Work out the finished part from the listing and answer in its coordinate system (mm). A direction names the side the tool comes from. Coordinates: 2 decimals unless noted, no trailing zeros. Order: outer loops, then holes, each group sorted by start corner. A loop starts at its lowest first (then second) coordinate and runs counter-clockwise, first axis right, second up.
1. A tool of negligible diameter and unlimited length cuts with its end or side. For faces 5 (the flat face through (10, -17, -17)), 6 (the cylindrical face through (18.11, 20.6, 12.68)), 7 (the flat face through (36, 2, -2)), from which of +Z, -Z, +X, -X, +Y, -Y can it reach the whole face along a straight path? Write none if from no direction.
2. Find the intervals of material crossed by probe 1 along Y at (x, z) = (33.5, 15.75); probe 2 along Z at (x, y) = (31, 15); probe 3 along X at (y, z) = (-17, -3.5), in increasing order.
3. Flat-ended cylindrical pins translate along their axes: pin 1 Ø4.5 at (y, z) = (-14.5, 15.5) entering from +X; pin 2 Ø2.5 at (x, z) = (44.5, 0) entering from +Y; pin 3 Ø1.8 at (y, z) = (15.75, 15.75) entering from +X. Find the tip coordinate at first contact, or state that the pin passes through.
4. The part is cut by section C-C, the plane x = 19.5. Give the vertices of the cut face in (y, z), then the cut area to 3 significant figures.
5. Determine the mould class of faces 1 (the cylindrical face through (32.06, -15.68, 17.25)), 2 (the flat face through (17.9, -16.8, -16.7)), 3 (the flat face through (28, -16, -16)), 4 (the cylindrical face through (18.11, -12.68, 20.6)) for opening direction Z: +Z half, -Z half, draft (parallel to the pull), parting line (faces both ways), or undercut.
6. The part is cut by section B-B, the plane z = 0. Give the vertices of the cut face in (x, y), then the cut area to 3 significant figures.
7. The part is cut by section A-A, the plane y = 15.75. Give the vertices of the cut face in (x, z), then the cut area to 3 significant figures.
Autodesk Inventor part; units mm, degrees
ref_plane "YZ Plane" through (0, 0, 0) normal (1, 0, 0) x (0, 1, 0)
ref_plane "XZ Plane" through (0, 0, 0) normal (0, 1, 0) x (-1, 0, 0)
ref_plane "XY Plane" through (0, 0, 0) normal (0, 0, 1) x (1, 0, 0)
sketch "Skizze2" plane through (0, 0, 0) normal (1, 0, 0) x (0, 1, 0)
  line L0 (20.75, -20.75) -> (-20.75, -20.75)
  line L1 (-20.75, -20.75) -> (-20.75, 20.75)
  line L2 (-20.75, 20.75) -> (20.75, 20.75)
  line L3 (20.75, 20.75) -> (20.75, -20.75)
  line L4 (-29.05, 0) -> (29.05, 0)
  line L5 (0, -29.05) -> (0, 29.05)
  point P0 (0, 0)
  dimension "d0" = 41.5
  dimension "d1" = 41.5
extrude "Extrusion1" add sketch "Skizze2" along normal blind 10
chamfer "Fase1" distance 3.5 angle 45 4 edges at (5, 20.75, 20.75) (5, 20.75, -20.75) (5, -20.75, -20.75) (5, -20.75, 20.75)
sketch "Skizze5" plane through (10, 0, 0) normal (1, 0, 0) x (0, 0, -1)
  line L0 (20.75, 20.75) -> (-20.75, 20.75)
  line L1 (-20.75, 20.75) -> (-20.75, -20.75)
  line L2 (-20.75, -20.75) -> (20.75, -20.75)
  line L3 (20.75, -20.75) -> (20.75, 20.75)
  line L4 (0, -29.064) -> (0, 29.1338)
  line L5 (17.25, 20.75) -> (-17.25, 20.75)
  line L6 (29.05, 0) -> (-29.05, 0)
  line L7 (20.75, -17.25) -> (20.75, 17.25)
  line L8 (20.75, 12.75) -> (12.75, 20.75)
  line L9 (17.25, 20.75) -> (20.75, 17.25)
  line L10 (-12.75, 20.75) -> (-20.75, 12.75)
  line L11 (-20.75, -12.75) -> (-12.75, -20.75)
  line L12 (12.75, -20.75) -> (20.75, -12.75)
  point P0 (0, 0)
  dimension "d11" = 41.5
  dimension "d12" = 41.5
  dimension "d20" = 8
  dimension "d21" = 8
  dimension "d24" = 360
extrude "Extrusion5" add sketch "Skizze5" along normal blind 16 contours L8 L3 L6 L4 L0 | L4 L6 L1 L10 L0 | L3 L12 L2 L4 L6 | L4 L2 L11 L1 L6
sketch "Skizze6" plane through (26, 0, 0) normal (1, 0, 0) x (0, 0, -1)
  line L0 (20.75, 20.75) -> (-20.75, 20.75)
  line L1 (-20.75, 20.75) -> (-20.75, -20.75)
  line L2 (-20.75, -20.75) -> (20.75, -20.75)
  line L3 (20.75, -20.75) -> (20.75, 20.75)
  line L4 (29.05, 0) -> (-29.05, 0)
  line L5 (0, -29.05) -> (0, 29.05)
  line L6 (20.75, 12.75) -> (20.75, 17.25)
  line L7 (20.75, 17.25) -> (17.25, 20.75)
  line L8 (-17.25, 20.75) -> (-20.75, 17.25)
  line L9 (-20.75, -17.25) -> (-17.25, -20.75)
  line L10 (17.25, -20.75) -> (20.75, -17.25)
  point P0 (0, 0)
  dimension "d28" = 41.5
  dimension "d29" = 41.5
  dimension "d32" = 360
extrude "Extrusion6" add sketch "Skizze6" along normal blind 10 contours L7 L3 L4 L5 L0 | L5 L4 L1 L8 L0 | L5 L2 L9 L1 L4 | L4 L3 L10 L2 L5
fillet "Rundung1" radius 2 8 edges at (18, 12.75, -20.75) (18, 20.75, -12.75) (18, -12.75, -20.75) (18, -20.75, -12.75) (18, -20.75, 12.75) (18, -12.75, 20.75) (18, 12.75, 20.75) (18, 20.75, 12.75)
sketch "Skizze7" plane through (36, 0, 0) normal (1, 0, 0) x (0, 0, -1)
  circle A0 centre (0, 0) radius 11.5
  circle A1 centre (15.75, -15.75) radius 1.5
  circle A2 centre (15.75, 15.75) radius 1.5
  circle A3 centre (-15.75, -15.75) radius 1.5
  circle A4 centre (-15.75, 15.75) radius 1.5
  dimension "d37" = 23
  dimension "d61" = 3
  dimension "d62" = 3
  dimension "d67" = 15.75
  dimension "d68" = 15.75
  dimension "d69" = 3
  dimension "d70" = 3
  dimension "d71" = 15.75
  dimension "d72" = 15.75
extrude "Extrusion7" add sketch "Skizze7" along normal blind 2 contours A0
sketch "Skizze8" plane through (38, 0, 0) normal (1, 0, 0) x (0, 0, -1)
  circle A0 centre (0, 0) radius 4
  dimension "d40" = 8
extrude "Extrusion8" cut sketch "Skizze8" against normal blind 2
sketch "Skizze9" plane through (36, 0, 0) normal (1, 0, 0) x (0, 0, -1)
  circle A0 centre (0, 0) radius 2.5
  line L0 (2.5, 0) -> (-2.5, 0)
  line L1 (-2.5, 0) -> (-2.5, 2.5)
  line L2 (-2.5, 2.5) -> (2.5, 2.5)
  line L3 (2.5, 2.5) -> (2.5, 0)
  line L4 (2.5, 2.5) -> (-2.5, 2.5)
  line L5 (-2.5, 2.5) -> (-2.5, 2)
  line L6 (-2.5, 2) -> (2.5, 2)
  line L7 (2.5, 2) -> (2.5, 2.5)
  point P0 (1.5, 2)
  point P1 (-1.5, 2)
  dimension "d43" = 5
  dimension "d44" = 0.5
  dimension "d47" = 2
extrude "Extrusion9" add sketch "Skizze9" along normal blind 20 contours L0 A0 | A0 L6 L0
sketch "Skizze10" plane through (0, -20.75, -17.25) normal (0, -1, 0) x (1, 0, 0)
  line L0 (0, 0) -> (0, 34.5)
  line L1 (0, 24.75) -> (10, 24.75)
  line L2 (10, 24.75) -> (10, 9.75)
  line L3 (10, 9.75) -> (0, 9.75)
  line L4 (0, 9.75) -> (0, 24.75)
  line L5 (0, 17.25) -> (36, 17.25)
  line L6 (36, 34.5) -> (36, 0)
  dimension "d48" = 10
  dimension "d49" = 15
extrude "Extrusion10" add sketch "Skizze10" along normal blind 4
extrude "Extrusion11" cut sketch "Skizze7" against normal blind 8 contours A1 | A2 | A3 | A4
properties part number "Steppermotor"
Geometry says:
1. face 5: -Z, -Y
1. face 6: +Z, +Y
1. face 7: +X
2. probe 1: y = -20.75 to -17.25, -14.25 to 14.25, 17.25 to 20.75
2. probe 2: z = -20.75 to -17.05, -14.45 to 14.45, 17.05 to 20.75
2. probe 3: x = 0 to 36
3. pin 1: stops at x = 36
3. pin 2: stops at y = 2
3. pin 3: stops at x = 28
4. outline: (-20.75, -11.92) arc R2 ccw to (-20.16, -13.34) - (-13.34, -20.16) arc R2 ccw to (-11.92, -20.75) - (11.92, -20.75) arc R2 ccw to (13.34, -20.16) - (20.16, -13.34) arc R2 ccw to (20.75, -11.92) - (20.75, 11.92) arc R2 ccw to (20.16, 13.34) - (13.34, 20.16) arc R2 ccw to (11.92, 20.75) - (-11.92, 20.75) arc R2 ccw to (-13.34, 20.16) - (-20.16, 13.34) arc R2 ccw to (-20.75, 11.92) - close
4. area: 1,590 mm2
5. face 1: undercut
5. face 2: -Z half
5. face 3: undercut
5. face 4: +Z half
6. outline: (0, -24.75) - (10, -24.75) - (10, -20.75) - (36, -20.75) - (36, -11.5) - (38, -11.5) - (38, -4) - (36, -4) - (36, -2.5) - (56, -2.5) - (56, 2) - (36, 2) - (36, 4) - (38, 4) - (38, 11.5) - (36, 11.5) - (36, 20.75) - (0, 20.75) - close
6. area: 1,650 mm2
7. outline: (0, -20.75) - (10, -20.75) - (10, -17.75) - (26, -17.75) - (26, -20.75) - (36, -20.75) - (36, -17.25) - (28, -17.25) - (28, -14.25) - (36, -14.25) - (36, 14.25) - (28, 14.25) - (28, 17.25) - (36, 17.25) - (36, 20.75) - (26, 20.75) - (26, 17.75) - (10, 17.75) - (10, 20.75) - (0, 20.75) - close
7. area: 1,350 mm2
